Read the model definition and answer for the solid it produces. Units are mm, in the model's axes. A direction names the side the tool comes from. Coordinates: 2 decimals unless noted, no trailing zeros. Loops run counter-clockwise (first coordinate to the right, second up) from the corner with the lowest first, then second, coordinate; pieces in that order, holes last. Notation, with made-up numbers: (-33.5, 63) -> (9.5, 63) arc R11 cw to (9.5, 79) -> close; hole circle Ø2 at (16.5, 28.25). An arc over 180 degrees is marked (long way). Answer as a JSON object with one key per item and string values. Group by question number.
1) Consider probe 1 along Y at (x, z) = (-50, 0.8); probe 2 along X at (y, z) = (35, 1.2); probe 3 along X at (y, z) = (22, 0.15). Determine where each line is inside the solid, lowest interval first. Write a range as [from, to].
2) Section A-A, the plane y = 0 is taken. Give the vertices of the cut face in (x, z).
3) Which of the six approach directions +Z, -Z, +X, -X, +Y, -Y give full straight-line access (tool end or side, diameter ignored) to faces 1 (the face through (25, 0, 1)), 2 (the face through (-60.918, -10.286, 0.986))?
4) Section B-B, the plane z = 1.7 is taken. Give the vertices of the cut face in (x, y).
5) Section C-C, the plane x = 50 is taken. Give the vertices of the cut face in (y, z).
6) Section D-D, the plane x = 14 is taken. Give the vertices of the cut face in (y, z), plus the area to 3 significant figures.
7) Determine the mould class of faces 3 (the face through (-1, 18, 0)), 4 (the face through (46.135, 29.329, 0.986)), 5 (the face through (-45.69, 29.9, 0.99)), 6 (the face through (-25, 0, 1)) for opening direction X: released by +X, released by -X, zero draft, split by the parting line, or undercut.
from build123d import *

# Parameters (mm, degrees)
F0_R     = 4
F1_DEPTH = 2


with BuildPart() as f1:
    # F0 (on Top) → F1 (new body)
    with BuildSketch(Plane.XY):
        with BuildLine():
            Line((-30, 50), (-61.824242, 9.229697))
            ThreePointArc((-61.824242, 9.229697), (-60.708366, -10.503852), (-41, -12))
            Line((-41, -12), (-9, 12))
            ThreePointArc((-9, 12), (0, 15), (9, 12))
            Line((9, 12), (41, -12))
            ThreePointArc((41, -12), (60.708366, -10.503852), (61.824242, 9.229697))
            Line((61.824242, 9.229697), (30, 50))
            Line((30, 50), (-30, 50))
        make_face()
        with Locations((-50, 0)):
            Circle(F0_R, mode=Mode.SUBTRACT)
        with Locations((50, 0)):
            Circle(F0_R, mode=Mode.SUBTRACT)
    extrude(amount=F1_DEPTH)


solid = f1.part
Determined:
{
 "1": {"probe 1": "[-15, -4], [4, 24.38]", "probe 2": "[-41.71, 41.71]", "probe 3": "[-51.86, 51.86]"},
 "2": {"outline": "(-65, 0) -> (-54, 0) -> (-54, 2) -> (-65, 2) -> close; (-46, 0) -> (-25, 0) -> (-25, 2) -> (-46, 2) -> close; (25, 0) -> (46, 0) -> (46, 2) -> (25, 2) -> close; (54, 0) -> (65, 0) -> (65, 2) -> (54, 2) -> close"},
 "3": {"face 1": "+Z, -Z, -Y", "face 2": "+Z, -Z"},
 "4": {"outline": "(-61.82, 9.23) arc R15 ccw to (-41, -12) -> (-9, 12) arc R15 cw to (9, 12) -> (41, -12) arc R15 ccw to (61.82, 9.23) -> (30, 50) -> (-30, 50) -> close; hole circle Ø8 at (-50, 0); hole circle Ø8 at (50, 0)"},
 "5": {"outline": "(-15, 0) -> (-4, 0) -> (-4, 2) -> (-15, 2) -> close; (4, 0) -> (24.38, 0) -> (24.38, 2) -> (4, 2) -> close"},
 "6": {"outline": "(8.25, 0) -> (50, 0) -> (50, 2) -> (8.25, 2) -> close", "area": "83.5 mm²"},
 "7": {"face 3": "zero draft", "face 4": "released by +X", "face 5": "released by -X", "face 6": "undercut"}
}
